Geometry: final body of the model. Coordinates: model frame, mm. Face numbers are marked on the shaded views. A direction names the side the tool comes from. Round coordinates to 2 decimals unless told otherwise and drop trailing zeros. Loops run counter-clockwise (first coordinate to the right, second up) from the corner with the lowest first, then second, coordinate; pieces in that order, holes last. Notation, with made-up numbers: M -35.5,42 L 17.5,42 A31 cw 17.5,72 Z; hole C 19,70.25 d9. An arc over 180 degrees is marked long. Answer as a JSON object with one key per item and string values.
Autodesk Inventor part; units mm, degrees
ref_plane "Work Plane2" through (3.35, 0, 0) normal (0, 0, -1) x (1, 0, 0)
ref_plane "YZ Plane" through (0, 0, 0) normal (1, 0, 0) x (0, 1, 0)
ref_plane "XZ Plane" through (0, 0, 0) normal (0, 1, 0) x (-1, 0, 0)
sketch "Sketch1" plane through (0, 0, 0) normal (0, 0, 1) x (1, 0, 0)
  line L0 (1.2, 0) -> (8, 0)
  line L1 (8, 0) -> (8, 1)
  line L2 (8, 1) -> (2, 1)
  line L3 (2, 1) -> (1.7546, 0.8773)
  line L4 (1.7546, 0.8773) -> (1.4071, 0.8773)
  line L5 (0, 1.9) -> (0, 0.95)
  line L6 (0, 0.95) -> (0.9455, 0.4786)
  line L7 (0.9455, 0.4786) -> (1.2, 0)
  line L8 (-1.6, 0) -> (9.6, 0)
  line L9 (0, -0.38) -> (0, 2.28)
  line L10 (0, 1.9) -> (0.1773, 1.9)
  line L11 (0.1773, 1.9) -> (1.0536, 1.0238)
  line L12 (2, 1) -> (1.0773, 1) construction
  arc A0 (1.0536, 1.0238) -> (1.4071, 0.8773) centre (1.4071, 1.3773) ccw
  point P0 (1.2, 0.8773)
  dimension "d1" = 6
  dimension "d2" = 2
  dimension "d3" = 1.7546
  dimension "d4" = 1.9
  dimension "d5" = 26.5
  dimension "d6" = 62
  dimension "d7" = 1.2
  dimension "d8" = 0.2454
  dimension "d12" = 3.8
  dimension "d13" = 45
  dimension "d15" = 8
  dimension "d24" = 1.2
  dimension "d93" = 0.5
revolve "Body" add sketch "Sketch1" angle 360 about axis through (1.2, 0, 0) along (1, 0, 0) contours L7 L6 L5 L10 L11 A0 L4 L3 L2 L1 L0
sketch "Sketch2" plane through (0, 0, 0) normal (-1, 0, 0) x (0, 0, 1)
  line L0 (0, 0.95) -> (0, 0) construction
  line L1 (0, 0) -> (0.95, 0) construction
  arc A0 (0.285, 0) -> (0, 0.285) centre (0, 0) ccw construction
  arc A1 (0.3325, 0) -> (0, 0.3325) centre (0, 0) ccw construction
  arc A2 (0.9373, 0.155) -> (0.155, 0.9373) centre (0, 0) ccw
  line L2 (0, 0) -> (0.6718, 0.6718) construction
  line L3 (0.155, 0.9373) -> (0.1646, 0.2889)
  line L4 (0.9373, 0.155) -> (0.2889, 0.1646)
  arc A3 (0.155, 0.9373) -> (0, 0.95) centre (0, 0) ccw
  arc A4 (0.95, 0) -> (0.9373, 0.155) centre (0, 0) ccw
  line L5 (0, -2.66) -> (0, 2.66)
  line L6 (-2.66, 0) -> (2.66, 0)
  arc A5 (0.155, -0.9373) -> (0.9373, -0.155) centre (0, 0) ccw
  line L7 (0.155, -0.9373) -> (0.1646, -0.2889)
  line L8 (0.9373, -0.155) -> (0.2889, -0.1646)
  arc A6 (0, -0.95) -> (0.155, -0.9373) centre (0, 0) ccw
  arc A7 (0.9373, -0.155) -> (0.95, 0) centre (0, 0) ccw
  arc A8 (-0.155, 0.9373) -> (-0.9373, 0.155) centre (0, 0) ccw
  line L9 (-0.155, 0.9373) -> (-0.1646, 0.2889)
  line L10 (-0.9373, 0.155) -> (-0.2889, 0.1646)
  arc A9 (0, 0.95) -> (-0.155, 0.9373) centre (0, 0) ccw
  arc A10 (-0.9373, 0.155) -> (-0.95, 0) centre (0, 0) ccw
  arc A11 (-0.155, -0.9373) -> (0, -0.95) centre (0, 0) ccw
  arc A12 (-0.9373, -0.155) -> (-0.155, -0.9373) centre (0, 0) ccw
  arc A13 (-0.95, 0) -> (-0.9373, -0.155) centre (0, 0) ccw
  line L11 (-0.9373, -0.155) -> (-0.2889, -0.1646)
  line L12 (-0.155, -0.9373) -> (-0.1646, -0.2889)
  arc A14 (0.1646, 0.2889) -> (0.2889, 0.1646) centre (0.2908, 0.2908) ccw
  arc A15 (0.2889, -0.1646) -> (0.1646, -0.2889) centre (0.2908, -0.2908) ccw
  arc A16 (-0.2889, 0.1646) -> (-0.1646, 0.2889) centre (-0.2908, 0.2908) ccw
  arc A17 (-0.1646, -0.2889) -> (-0.2889, -0.1646) centre (-0.2908, -0.2908) ccw
  point P0 (0.6718, -0.6718)
  point P1 (-0.6718, 0.6718)
  point P2 (-0.6718, -0.6718)
  dimension "d17" = 0.57
  dimension "d18" = 0.665
  dimension "d19" = 1.9
  dimension "d20" = 45
  dimension "d21" = 0.155
extrude "Slot" add sketch "Sketch2" against normal up to next draft 5 contours L4 A14 L3 A2 | A5 L7 A15 L8 | L9 A16 L10 A8 | A12 L11 A17 L12
fillet "Fillet1" radius 0.062 4 edges at (0, 0.95, 0) (0, 0, -0.95) (0, -0.95, 0) (0, 0, 0.95)
thread "Thread"
chamfer "Chamfer1" distance 0.2454 distance2 0.1227 1 edges at (8, -1, 0) measured on face at (8, -0.1182, -0.3117)
ref_plane "Work Plane2" through (3.35, 0, 0) normal (0, 0, -1) x (1, 0, 0)
equation "\"d1\" = GEL"
equation "\"d2\" = GD"
equation "\"d3\" = BDM"
equation "\"d4\" = SDM"
equation "\"d7\" = INTI"
equation "\"d8\" = GAL"
equation "\"d12\" = KOD"
equation "\"d13\" = 0.5 * SEWI"
equation "\"d15\" = NLG"
equation "\"d93\" = R"
equation "\"d17\" = 0.3 * SDM"
equation "\"d18\" = 0.35 * SDM"
equation "\"d19\" = SDM"
equation "\"d21\" = 0.5 * SBR"
equation "\"d23\" = 0.2 * SBR"
equation "\"d10\" = GEL"
equation "\"d25\" = -0.5 * SPD + 0.5 * GD"
equation "\"d26\" = 0.5 * GAL"
equation "\"NLG\" = 8"
equation "\"GEL\" = 6"
equation "\"GAL\" = 0.61345 * PTC"
equation "\"SPD\" = NND - 1.2269 * PTC"
equation "\"KOD\" = 3.8"
equation "\"KOH\" = 1.2"
equation "\"SBR\" = 0.31"
equation "\"INTI\" = 1.2"
equation "\"SDM\" = 1.9"
equation "\"GD\" = NND"
equation "\"BDM\" = NND - GAL"
equation "\"SEWI\" = 90deg"
equation "\"d9\" = SDM"
equation "\"R\" = 0.5"
equation "\"GUL\" = 0.61345 * PTC"
equation "\"TOA\" = 30deg"
equation "\"EPV\" = 2.2"
equation "\"THREADDIA\" = 2"
equation "\"PTC\" = 0.4"
equation "\"NND\" = 2"
equation "\"GD1\" = THREADDIA - 1.2269 * PTC"
properties part number "ISO 7046-1  - M2 x 8 - 4.8 - H" material "Steel"
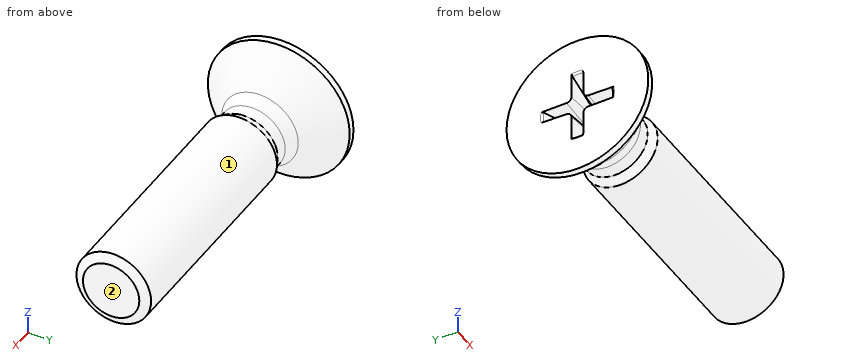
1) Ray query, line 1 (Y direction, x = 6.75, z = 0.15); line 2 (Z direction, x = 4.5, y = 0.05); line 3 (X direction, y = 0.75, z = -1.7). Return the intervals inside material, ascending.
Results:
{"line 1": "-0.99 to 0.99", "line 2": "-1 to 1", "line 3": "0 to 0.22"}
2) Reachability of the marked faces 1 and 2 from +Z, -Z, +X, -X, +Y, -Y: full face, straight path, thin tool, end or side. Return the list, or none.
Results:
{"face 1": "+X", "face 2": "+Z, -Z, +X, +Y, -Y"}
3) Section query B-B (x = 1.5). Return the cut outline in (y, z).
Results:
{"outline": "C 0,0 d1.75"}
4) Section query A-A (x = 2.5). Return the cut outline in (y, z), and give its area (3 significant figures).
Results:
{"outline": "C 0,0 d2", "area": "3.14 mm2"}
